```python
from build123d import *

# Parameters (mm, degrees)
BOSS_EXTRUDE1_DEPTH = 50.8
CUT_EXTRUDE1_REACH  = 138.783
SKETCH2_R           = 4.7625
SKETCH3_R           = 19.05
BOSS_EXTRUDE2_DEPTH = 3.175
FILLET1_R           = 6.35
FILLET2_R           = 3.175
CHAMFER1_SIZE       = 6.35


with BuildPart() as part:
    # Sketch1 → Boss-Extrude1 (new, symmetric)
    with BuildSketch(Plane.XY):
        Polygon((34.925, 76.2), (63.5, 76.2), (63.5, 88.9), (101.6, 88.9), (101.6, 0), (-101.6, 0), (-101.6, 88.9), (-63.5, 88.9), (-63.5, 76.2), (-34.925, 76.2), (-34.925, 63.5), (-76.2, 63.5), (-76.2, 76.2), (-88.9, 76.2), (-88.9, 12.7), (88.9, 12.7), (88.9, 76.2), (76.2, 76.2), (76.2, 63.5), (34.925, 63.5), align=None)
    extrude(amount=BOSS_EXTRUDE1_DEPTH, both=True)

    # Sketch2 → Cut-Extrude1 (cut, up to next)
    with BuildSketch(Plane(origin=(0, 76.2, 0), x_dir=(1, 0, 0), z_dir=(0, 1, 0)), mode=Mode.PRIVATE) as cut_extrude1_sk1:
        with Locations(Location((-50.8, 19.05, 0), (0, 0, 270))):
            Circle(SKETCH2_R)
    cut_extrude1_tool1 = extrude(cut_extrude1_sk1.sketch, amount=-CUT_EXTRUDE1_REACH, mode=Mode.PRIVATE) & part.part
    # Sketch2 → Cut-Extrude1 (cut, up to next)
    with BuildSketch(Plane(origin=(0, 76.2, 0), x_dir=(1, 0, 0), z_dir=(0, 1, 0)), mode=Mode.PRIVATE) as cut_extrude1_sk2:
        with Locations(Location((-50.8, -19.05, 0), (0, 0, 270))):
            Circle(SKETCH2_R)
    cut_extrude1_tool2 = extrude(cut_extrude1_sk2.sketch, amount=-CUT_EXTRUDE1_REACH, mode=Mode.PRIVATE) & part.part
    # Sketch2 → Cut-Extrude1 (cut, up to next)
    with BuildSketch(Plane(origin=(0, 76.2, 0), x_dir=(1, 0, 0), z_dir=(0, 1, 0)), mode=Mode.PRIVATE) as cut_extrude1_sk3:
        with Locations(Location((50.8, 19.05, 0), (0, 0, 270))):
            Circle(SKETCH2_R)
    cut_extrude1_tool3 = extrude(cut_extrude1_sk3.sketch, amount=-CUT_EXTRUDE1_REACH, mode=Mode.PRIVATE) & part.part
    # Sketch2 → Cut-Extrude1 (cut, up to next)
    with BuildSketch(Plane(origin=(0, 76.2, 0), x_dir=(1, 0, 0), z_dir=(0, 1, 0)), mode=Mode.PRIVATE) as cut_extrude1_sk4:
        with Locations(Location((50.8, -19.05, 0), (0, 0, 270))):
            Circle(SKETCH2_R)
    cut_extrude1_tool4 = extrude(cut_extrude1_sk4.sketch, amount=-CUT_EXTRUDE1_REACH, mode=Mode.PRIVATE) & part.part
    add(cut_extrude1_tool1.solids().sort_by_distance((-50.8, 76.2, -19.05))[0], mode=Mode.SUBTRACT)
    add(cut_extrude1_tool2.solids().sort_by_distance((-50.8, 76.2, 19.05))[0], mode=Mode.SUBTRACT)
    add(cut_extrude1_tool3.solids().sort_by_distance((50.8, 76.2, -19.05))[0], mode=Mode.SUBTRACT)
    add(cut_extrude1_tool4.solids().sort_by_distance((50.8, 76.2, 19.05))[0], mode=Mode.SUBTRACT)

    # Sketch3 → Boss-Extrude2 (add, symmetric)
    with BuildSketch(Plane(origin=(0, 12.7, 0), x_dir=(1, 0, 0), z_dir=(0, 1, 0))):
        Circle(SKETCH3_R)
    extrude(amount=BOSS_EXTRUDE2_DEPTH, both=True)

    # Fillet1
    fillet1_edges = [part.edges().sort_by_distance(p)[0] for p in [
        (-88.9, 12.7, 0),
        (88.9, 12.7, 0),
    ]]
    fillet(fillet1_edges, radius=FILLET1_R)

    # Fillet2
    fillet2_edges = [part.edges().sort_by_distance(p)[0] for p in [
        (-19.05, 12.7, 0),
    ]]
    fillet(fillet2_edges, radius=FILLET2_R - 0.0001)  # a hair under: the kernel refuses the full size

    # Chamfer1
    chamfer1_edges = [part.edges().sort_by_distance(p)[0] for p in [
        (63.5, 88.9, 0),
        (-63.5, 88.9, 0),
    ]]
    chamfer(chamfer1_edges, length=CHAMFER1_SIZE)


solid = part.part
```
Read the model definition and answer for the solid it produces. Units are mm, in the model's axes. A direction names the side the tool comes from. Round coordinates to 2 decimals unless told otherwise and drop trailing zeros. Write each loop counter-clockwise with the first axis right and the second up, starting at its lowest first coordinate (ties: lowest second). Pieces come first, ordered by that corner, then holes. Notation, with made-up numbers: (51.25, 61) -> (63.25, 61) arc R23 ccw to (63.25, 77) -> close; hole circle Ø10 at (-34.75, -33.75). An arc over 180 degrees is marked (long way). Answer in a Markdown table with one row per item. Add a question column.
1) Find section D-D, the plane z = -36. Determine the outline of the cut face in (x, y) (3 decimals), and give its area (3 significant figures).
2) Consider line 1 (X direction, y = 69, z = 31) (3 decimals); line 2 (X direction, y = 72.5, z = 19.05) (1 decimal); line 3 (Y direction, x = -40.5, z = 33). Determine where each line is inside the solid, lowest interval first.
3) Given P1, Ø11, axis at x = -50.8, z = -19.05, coming from the +Y side; P2, Ø4, axis at x = -25.5, z = 37, coming from the +Y side; P3, Ø19, axis at x = -9, z = -0.5, coming from the +Y side (3 decimals), each flat-ended and moving along its own axis, determine where each tip first touches the part or whether it passes through.
4) Find section B-B, the plane x = 50.8. Determine the outline of the cut face in (y, z), and give its area (3 significant figures).
5) Find section A-A, the plane y = 45.5. Determine the outline of the cut face in (x, z).
6) Which of the six approach directions +Z, -Z, +X, -X, +Y, -Y give full straight-line access (tool end or side, diameter ignored) to faces 5 (the face through (49, 76.2, 1)), 6 (the face through (-55, 63.5, 1)), 7 (the face through (52.2, 69.9, -14.5)), 8 (the face through (101.6, 45, 1)), 9 (the face through (-86, 88.9, 1))?
7) Determine the mould class of faces 1 (the face through (1, 0, 1)), 2 (the face through (-66.72, 85.77, 0.71)), 3 (the face through (56, 63.5, 1)), 4 (the face through (-101.6, 44, 1)) for opening direction Y: pulls with the +Y half, pulls with the -Y half, needs draft (parallel to the pull), parting line crosses it, or undercut.
Findings below:
| question | item | result |
|---|---|---|
| 1 | outline | (-101.6, 0) -> (101.6, 0) -> (101.6, 88.9) -> (69.85, 88.9) -> (63.5, 82.55) -> (63.5, 76.2) -> (34.925, 76.2) -> (34.925, 63.5) -> (76.2, 63.5) -> (76.2, 76.2) -> (88.9, 76.2) -> (88.9, 19.05) arc R6.35 cw to (82.55, 12.7) -> (-82.55, 12.7) arc R6.35 cw to (-88.9, 19.05) -> (-88.9, 76.2) -> (-76.2, 76.2) -> (-76.2, 63.5) -> (-34.925, 63.5) -> (-34.925, 76.2) -> (-63.5, 76.2) -> (-63.5, 82.55) -> (-69.85, 88.9) -> (-101.6, 88.9) -> close |
| 1 | area | 6,190 mm² |
| 2 | line 1 | -101.6 to -88.9, -76.2 to -34.925, 34.925 to 76.2, 88.9 to 101.6 |
| 2 | line 2 | -101.6 to -88.9, -76.2 to -55.6, -46 to -34.9, 34.9 to 46, 55.6 to 76.2, 88.9 to 101.6 |
| 2 | line 3 | 0 to 12.7, 63.5 to 76.2 |
| 3 | P1 | y = 76.2 |
| 3 | P2 | y = 12.7 |
| 3 | P3 | y = 15.875 |
| 4 | outline | (0, -50.8) -> (12.7, -50.8) -> (12.7, 50.8) -> (0, 50.8) -> close; (63.5, -50.8) -> (76.2, -50.8) -> (76.2, -23.81) -> (63.5, -23.81) -> close; (63.5, -14.29) -> (76.2, -14.29) -> (76.2, 14.29) -> (63.5, 14.29) -> close; (63.5, 23.81) -> (76.2, 23.81) -> (76.2, 50.8) -> (63.5, 50.8) -> close |
| 4 | area | 2,340 mm² |
| 5 | outline | (-101.6, -50.8) -> (-88.9, -50.8) -> (-88.9, 50.8) -> (-101.6, 50.8) -> close; (88.9, -50.8) -> (101.6, -50.8) -> (101.6, 50.8) -> (88.9, 50.8) -> close |
| 6 | face 5 | +Z, -Z, +Y |
| 6 | face 6 | +Z, -Z |
| 6 | face 7 | +Y |
| 6 | face 8 | +Z, -Z, +X, +Y, -Y |
| 6 | face 9 | +Z, -Z, +X, -X, +Y |
| 7 | face 1 | pulls with the -Y half |
| 7 | face 2 | pulls with the +Y half |
| 7 | face 3 | undercut |
| 7 | face 4 | needs draft |
